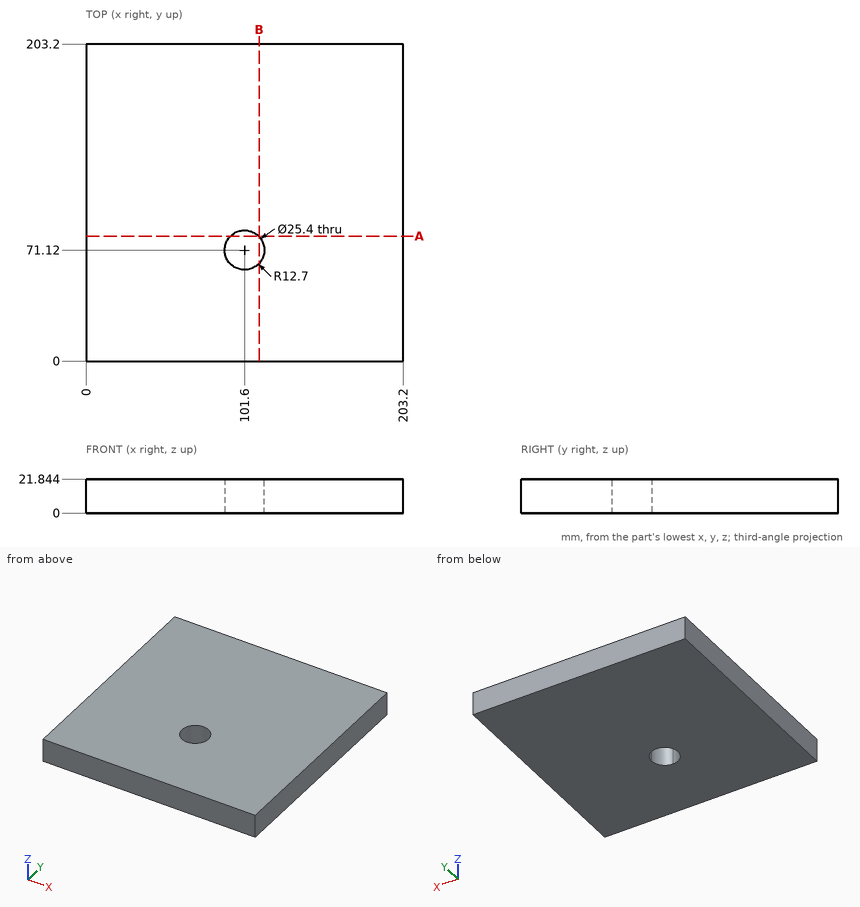
Source: three-view drawing plus pictorial views. Frame: mm from the lowest corner of the part. Coordinates: 2 decimals unless noted, no trailing zeros. Write each loop counter-clockwise with the first axis right and the second up, starting at its lowest first coordinate (ties: lowest second). Pieces come first, ordered by that corner, then holes. Notation, with made-up numbers: (-15, -1) - (15, -1) arc R13 ccw to (15, 8) - close; hole circle Ø10 at (61.25, 38.25). An arc over 180 degrees is marked (long way). Answer as a JSON object with one key per item and string values.
Q1. Material intervals for line 1 (Y direction, x = 101.6, z = 14.5); line 2 (X direction, y = 71.12, z = 6.5); line 3 (Y direction, x = 91, z = 11.5) (3 decimals), sorted ascending. Write a range as [from, to].
Ans:
{"line 1": "y = [0, 58.42], [83.82, 203.2]", "line 2": "x = [0, 88.9], [114.3, 203.2]", "line 3": "y = [0, 64.125], [78.115, 203.2]"}
Q2. Section query B-B, the plane x = 111. Output: boundary loops of the cut face in (y, z), plus the area to 3 significant figures.
Ans:
{"outline": "(0, 0) - (62.58, 0) - (62.58, 21.84) - (0, 21.84) - close; (79.66, 0) - (203.2, 0) - (203.2, 21.84) - (79.66, 21.84) - close", "area": "4,070 mm2"}
Q3. Section query A-A, the plane y = 80. Output: boundary loops of the cut face in (x, z), plus the area to 3 significant figures.
Ans:
{"outline": "(0, 0) - (92.52, 0) - (92.52, 21.84) - (0, 21.84) - close; (110.68, 0) - (203.2, 0) - (203.2, 21.84) - (110.68, 21.84) - close", "area": "4,040 mm2"}
